For this review, use the dimensioned drawing (mm, ordinates from the lowest corner) and the shaded views. A direction names the side the tool comes from. Give positions to 0.01 mm unless a question says otherwise; leave off trailing zeros. Write each loop counter-clockwise with the first axis right and the second up, starting at its lowest first coordinate (ties: lowest second). Pieces come first, ordered by that corner, then holes. Notation, with made-up numbers: M 50,-1.5 L 75,-1.5 A14 ccw 75,7.5 Z; hole C 26,72 d4. An arc over 180 degrees is marked long. Answer in a Markdown table with one row per item.
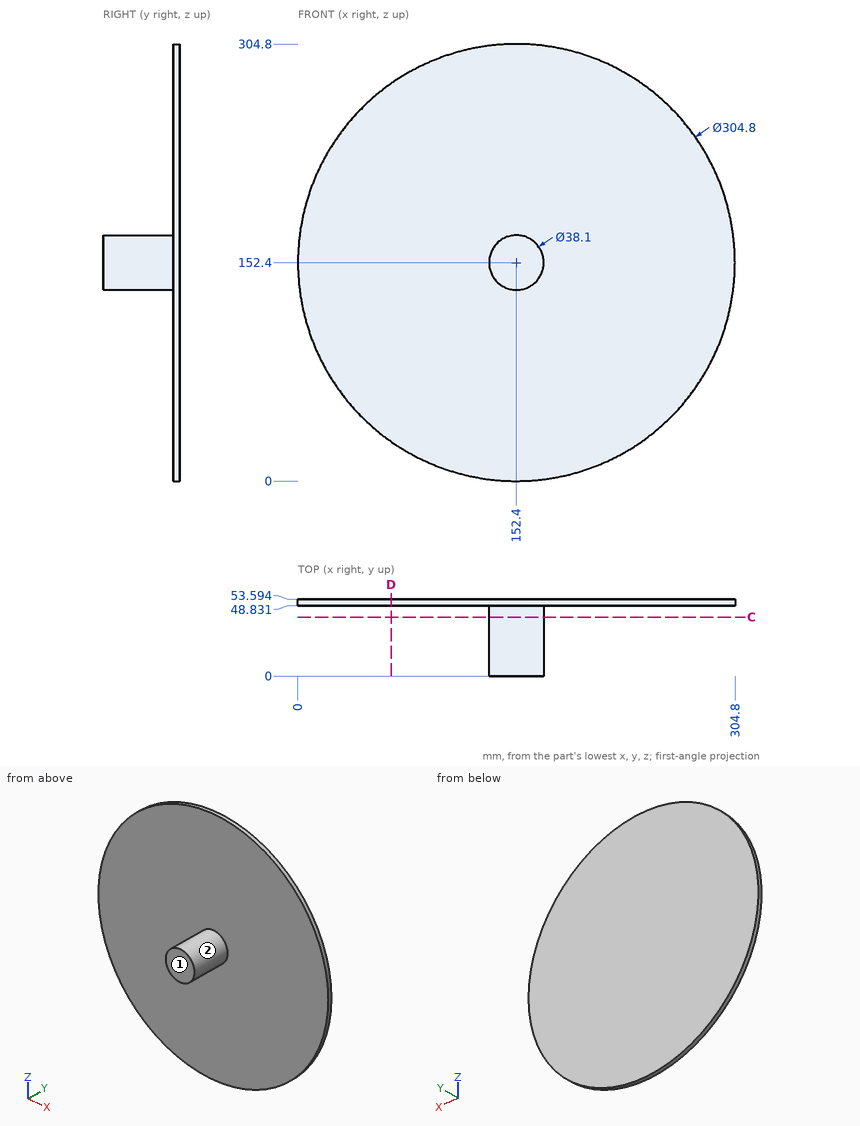
1) Add section D-D (x = 65). Write out the cut boundary in (y, z) (1 decimal).
Geometry says:
| item | result |
|---|---|
| outline | M 48.8,27.6 L 53.6,27.6 L 53.6,277.2 L 48.8,277.2 Z |
2) Insertion check: P1, Ø10, axis at x = 48, z = 237, coming from the -Y side; P2, Ø1, axis at y = 39.5, z = 165, coming from the -X side (1 decimal). Each pin has a flat end and moves straight along its axis. Give the tip position at first contact, or say it passes through.
Geometry says:
| item | result |
|---|---|
| P1 | y = 48.83 |
| P2 | x = 137.7 |
3) To check wall thickness, follow probe 1 along Y at (x, z) = (255, 150.5) (1 decimal); probe 2 along Z at (x, y) = (218.5, 51); probe 3 along X at (y, z) = (51.5, 146.5) (1 decimal). State the ranges of each line that lie inside material, in increasing order. Write a range as [from, to].
Geometry says:
| item | result |
|---|---|
| probe 1 | [48.8, 53.6] |
| probe 2 | [15.08, 289.72] |
| probe 3 | [0.1, 304.7] |
4) Add section C-C (y = 41). Write out the cut boundary in (x, z).
Geometry says:
| item | result |
|---|---|
| outline | C 152.4,152.4 d38.1 |
5) For the marked faces 1 and 2, list the 3-axis set-ups (+Z, -Z, +X, -X, +Y, -Y) from which the entire face can be reached by the end or side of a thin tool; tool diameter is ignored.
Geometry says:
| item | result |
|---|---|
| face 1 | +Z, -Z, +X, -X, -Y |
| face 2 | -Y |
